```python
from build123d import *

# Parameters (mm, degrees)
SKETCH_1_R      = 3
EXTRUDE_1_DEPTH = 6
SKETCH_2_R      = 18.5
SKETCH_2_R_2    = 14.5
EXTRUDE_2_DEPTH = 6
FILLET_1_R      = 2
CHAMFER_1_SIZE  = 0.5


with BuildPart() as part:
    # 草图1 → 凸台-拉伸1 (new body)
    with BuildSketch(Plane(origin=(0, 0, 0), x_dir=(1, 0, 0), z_dir=(0, 1, 0))):
        with BuildLine():
            Line((-14.422205102, 24), (14.422205102, 24))
            ThreePointArc((14.422205102, 24), (0, -28), (-14.422205102, 24))
        make_face()
        with Locations(Location((-16.263455967, 16.263455967, 0), (0, 0, 270))):
            Circle(SKETCH_1_R, mode=Mode.SUBTRACT)
        with Locations(Location((16.263455967, 16.263455967, 0), (0, 0, 270))):
            Circle(SKETCH_1_R, mode=Mode.SUBTRACT)
        with Locations(Location((16.263455967, -16.263455967, 0), (0, 0, 270))):
            Circle(SKETCH_1_R, mode=Mode.SUBTRACT)
        with Locations(Location((-16.263455967, -16.263455967, 0), (0, 0, 270))):
            Circle(SKETCH_1_R, mode=Mode.SUBTRACT)
    extrude(amount=EXTRUDE_1_DEPTH)

    # 草图2 → 凸台-拉伸2 (add)
    with BuildSketch(Plane(origin=(0, 6, 0), x_dir=(1, 0, 0), z_dir=(0, 1, 0))):
        with Locations(Location((0, 0, 0), (0, 0, 270))):
            Circle(SKETCH_2_R)
        with Locations(Location((0, 0, 0), (0, 0, 270))):
            Circle(SKETCH_2_R_2, mode=Mode.SUBTRACT)
    extrude(amount=EXTRUDE_2_DEPTH)

    # 圆角1
    fillet_1_edges = [part.edges().sort_by_distance(p)[0] for p in [
        (0, 0, 28),
    ]]
    fillet(fillet_1_edges, radius=FILLET_1_R - 0.0001)  # a hair under: the kernel refuses the full size

    # 倒角1
    chamfer_1_edges = [part.edges().sort_by_distance(p)[0] for p in [
        (0, 12, -18.5),
    ]]
    chamfer(chamfer_1_edges, length=CHAMFER_1_SIZE)


solid = part.part
```
Input: part model. Units: mm. Frame: model coordinates. A direction names the side the tool comes from. Coordinates: 2 decimals unless noted, no trailing zeros. Loops run counter-clockwise (first coordinate to the right, second up) from the corner with the lowest first, then second, coordinate; pieces in that order, holes last. Notation, with made-up numbers: M 78,41 L 129,41 A10 ccw 129,58 Z; hole C 53.25,76 d8. An arc over 180 degrees is marked long. Answer in a Markdown table with one row per item.
1. Reachability of faces 4 (the flat face through (0, 6, 0)), 5 (the flat face through (0, 0, 1)) from +Z, -Z, +X, -X, +Y, -Y: full face, straight path, thin tool, end or side. Return the list, or none.
Response:
| item | result |
|---|---|
| face 4 | +Y |
| face 5 | +Z, -Z, +X, -X, -Y |
2. Section B-B, the plane y = 3.25. Output: boundary loops of the cut face in (x, z).
Response:
| item | result |
|---|---|
| outline | M -14.42,-24 L 14.42,-24 A28 ccw long Z; hole C -16.26,-16.26 d6; hole C -16.26,16.26 d6; hole C 16.26,-16.26 d6; hole C 16.26,16.26 d6 |
3. Material intervals for line 1 (Z direction, x = 18, y = 2); line 2 (X direction, y = 5, z = -17.5); line 3 (Z direction, x = 19, y = 5.25), sorted ascending.
Response:
| item | result |
|---|---|
| line 1 | z = -21.45 to -18.71, -13.82 to 13.82, 18.71 to 21.45 |
| line 2 | x = -21.86 to -19, -13.53 to 13.53, 19 to 21.86 |
| line 3 | z = -20.57 to -17.49, -15.03 to 15.03, 17.49 to 20.57 |
4. Section C-C, the plane y = 10. Output: boundary loops of the cut face in (x, z), then the cut area to 3 significant figures.
Response:
| item | result |
|---|---|
| outline | C 0,0 d37; hole C 0,0 d29 |
| area | 415 mm2 |
5. Draft query along Z for faces 1 (the flat face through (0, 6, 19)), 2 (the cylindrical face through (-17.412, 2.958, 19.035)), 3 (the cylindrical face through (-7.086, 8.712, 17.089)). Return one class per face: pulls with the +Z half, pulls with the -Z half, needs draft (parallel to the pull), parting line crosses it, or undercut.
Response:
| item | result |
|---|---|
| face 1 | needs draft |
| face 2 | undercut |
| face 3 | parting line crosses it |
6. First-contact query: pin 1 (1 mm diameter, centred on x = 22, z = 10.5, fed in from +Y); pin 2 (1.5 mm diameter, centred on y = 7.5, z = 1.5, fed in from +X); pin 3 (2 mm diameter, centred on y = 6.5, z = -11, fed in from +X); pin 4 (5.5 mm diameter, centred on x = -16.26, z = -16.26, fed in from +Y). Flat tips, straight axial feed; report the tip coordinate or a pass-through.
Response:
| item | result |
|---|---|
| pin 1 | stops at y = 6 |
| pin 2 | stops at x = 18.48 |
| pin 3 | stops at x = 26.1 |
| pin 4 | passes through |
7. Section A-A, the plane x = 0. Output: boundary loops of the cut face in (y, z).
Response:
| item | result |
|---|---|
| outline | M 0,-24 L 6,-24 L 6,-18.5 L 11.5,-18.5 L 12,-18 L 12,-14.5 L 6,-14.5 L 6,14.5 L 12,14.5 L 12,18 L 11.5,18.5 L 6,18.5 L 6,28 L 2,28 A2 ccw 0,26 Z |
